Can you work these out from the model? Positions are in its coordinate system, mm. A direction names the side the tool comes from. Give positions to 0.01 mm unless a question says otherwise; leave off trailing zeros. Loops run counter-clockwise (first coordinate to the right, second up) from the corner with the lowest first, then second, coordinate; pieces in that order, holes last. Notation, with made-up numbers: M -29,20.5 L 14,20.5 A30 ccw 14,43.5 Z; hole C 5,-32 d11. An arc over 180 degrees is marked long. Answer as a JSON object with one key per item and string values.
```python
from build123d import *

# Parameters (mm, degrees)
SKETCH1_R           = 4.7625
BOSS_EXTRUDE1_DEPTH = 6.35


with BuildPart() as part:
    # Sketch1 → Boss-Extrude1 (new body)
    with BuildSketch(Plane(origin=(0, 0, 0), x_dir=(1, 0, 0), z_dir=(0, 1, 0))):
        with BuildLine():
            Line((0, 132.63), (0, 28.05))
            ThreePointArc((0, 28.05), (-2.636038969, 21.686038969), (-9, 19.05))
            Line((-9, 19.05), (-9.525, 19.05))
            ThreePointArc((-9.525, 19.05), (-19.05, 9.525), (-9.525, 0))
            Line((-9.525, 0), (0, 0))
            Line((0, 0), (77, 0))
            Line((77, 0), (86.525, 0))
            ThreePointArc((86.525, 0), (96.05, 9.525), (86.525, 19.05))
            Line((86.525, 19.05), (86, 19.05))
            ThreePointArc((86, 19.05), (79.636038969, 21.686038969), (77, 28.05))
            Line((77, 28.05), (77, 132.63))
            ThreePointArc((77, 132.63), (79.636038969, 138.993961031), (86, 141.63))
            Line((86, 141.63), (86.525, 141.63))
            ThreePointArc((86.525, 141.63), (96.05, 151.155), (86.525, 160.68))
            Line((86.525, 160.68), (86, 160.68))
            ThreePointArc((86, 160.68), (79.636038969, 163.316038969), (77, 169.68))
            Line((77, 169.68), (77, 172))
            ThreePointArc((77, 172), (74.363961031, 178.363961031), (68, 181))
            Line((68, 181), (9, 181))
            ThreePointArc((9, 181), (2.636038969, 178.363961031), (0, 172))
            Line((0, 172), (0, 169.68))
            ThreePointArc((0, 169.68), (-2.636038969, 163.316038969), (-9, 160.68))
            Line((-9, 160.68), (-9.525, 160.68))
            ThreePointArc((-9.525, 160.68), (-19.05, 151.155), (-9.525, 141.63))
            Line((-9.525, 141.63), (-9, 141.63))
            ThreePointArc((-9, 141.63), (-2.636038969, 138.993961031), (0, 132.63))
        make_face()
        with Locations((86.525, 151.155)):
            Circle(SKETCH1_R, mode=Mode.SUBTRACT)
        with Locations((-9.525, 151.155)):
            Circle(SKETCH1_R, mode=Mode.SUBTRACT)
        with Locations((-9.525, 9.525)):
            Circle(SKETCH1_R, mode=Mode.SUBTRACT)
        with Locations((86.525, 9.525)):
            Circle(SKETCH1_R, mode=Mode.SUBTRACT)
    extrude(amount=BOSS_EXTRUDE1_DEPTH)


solid = part.part
```
1) For faces 1 (the cylindrical face through (79.706, 3.131, -163.246)), 2 (the cylindrical face through (-2.566, 3.131, -21.756)), 3 (the cylindrical face through (79.706, 3.131, -21.616)), which set-ups out of +Z, -Z, +X, -X, +Y, -Y let a thin tool reach every point of the face, with its end or its side?
Answer list:
{"face 1": "-Z, +X, +Y, -Y", "face 2": "-X, +Y, -Y", "face 3": "+X, +Y, -Y"}
2) Suppose I cut it at D-D, the plane z = -164. Write out the boundary of the cut face in (x, y).
Answer list:
{"outline": "M -2.02,0 L 79.02,0 L 79.02,6.35 L -2.02,6.35 Z"}
3) Suppose I cut it at A-A, the plane x = -12. Write out the boundary of the cut face in (y, z), and give its area (3 significant figures).
Answer list:
{"outline": "M 0,-160.35 L 6.35,-160.35 L 6.35,-155.22 L 0,-155.22 Z; M 0,-147.09 L 6.35,-147.09 L 6.35,-141.96 L 0,-141.96 Z; M 0,-18.72 L 6.35,-18.72 L 6.35,-13.59 L 0,-13.59 Z; M 0,-5.46 L 6.35,-5.46 L 6.35,-0.33 L 0,-0.33 Z", "area": "130 mm^2"}
4) If we mould it in two halves opening along Z, with no side actions, what happens to faces 4 (the flat face through (39, 3, -181)), 5 (the cylindrical face through (-19.048, 3.131, -151.364)), 6 (the flat face through (38, 3, 0))? For each: +Z half, -Z half, draft (parallel to the pull), parting line (faces both ways), or undercut.
Answer list:
{"face 4": "-Z half", "face 5": "undercut", "face 6": "+Z half"}
5) Will these pins go through, and if not, where does the flat tip stop? pin 1 Ø1.5 at (y, z) = (4, -113) entering from -X; pin 2 Ø5.5 at (x, z) = (86.525, -9.525) entering from -Y; pin 3 Ø2 at (x, y) = (37.5, 5) entering from +Z; pin 4 Ø3 at (y, z) = (4, -81) entering from +X.
Answer list:
{"pin 1": "x = 0", "pin 2": "through", "pin 3": "z = 0", "pin 4": "x = 77"}
6) Please list where these lines run through material, in increasing order: line 1 along Z through (x, y) = (90.5, 0.75); line 2 along Z through (x, y) = (90, 3.5); line 3 along X through (y, z) = (3.5, -94). Write a range as from..to.
Answer list:
{"line 1": "-159.81..-153.78, -148.53..-142.5, -18.18..-12.15, -6.9..-0.87", "line 2": "-160.02..-154.41, -147.9..-142.29, -18.39..-12.78, -6.27..-0.66", "line 3": "0..77"}
7) Suppose I cut it at C-C, the plane z = -98. Write out the boundary of the cut face in (x, y), and give its area (3 significant figures).
Answer list:
{"outline": "M 0,0 L 77,0 L 77,6.35 L 0,6.35 Z", "area": "489 mm^2"}
8) Suppose I cut it at B-B, the plane y = 4. Give the number of separate pieces and of enclosed holes in the cut face, and give its area (3 significant figures).
Answer list:
{"separate pieces": "1", "enclosed holes": "4", "area": "15,000 mm^2"}
